Design review of the part built by this model. Coordinates are the model's own, in mm. A direction names the side the tool comes from. Give positions to 0.01 mm unless a question says otherwise; leave off trailing zeros. Write each loop counter-clockwise with the first axis right and the second up, starting at its lowest first coordinate (ties: lowest second). Pieces come first, ordered by that corner, then holes. Notation, with made-up numbers: (85, 67.5) -> (91, 67.5) arc R36 cw to (91, 105.5) -> close; hole circle Ø9 at (37.5, 78). An arc over 180 degrees is marked (long way). Answer as a JSON object with one key per item and string values.
```python
from build123d import *

# Parameters (mm, degrees)
EXTRUDE_1_DEPTH     = 3
SKETCH_2_R          = 1.65
CUT_EXTRUDE_1_DEPTH = 4
SKETCH_3_W          = 40
SKETCH_3_H          = 3
EXTRUDE_2_DEPTH     = 20
EXTRUDE_3_DEPTH     = 1.5


with BuildPart() as part:
    # 草图1 → 凸台-拉伸1 (new body)
    with BuildSketch(Plane(origin=(0, 0, 0), x_dir=(0, 0, -1), z_dir=(1, 0, 0))):
        with BuildLine():
            Line((-20, 0), (20, 0))
            Line((20, 0), (20, 3))
            Line((20, 3), (7.638784068, 24.410254038))
            ThreePointArc((7.638784068, 24.410254038), (0, 28.820508076), (-7.638784068, 24.410254038))
            Line((-7.638784068, 24.410254038), (-20, 3))
            Line((-20, 3), (-20, 0))
        make_face()
    extrude(amount=-EXTRUDE_1_DEPTH)

    # 草图2 → 切除-拉伸1 (cut, through all)
    with BuildSketch(Plane(origin=(0, 0, 0), x_dir=(0, 0, -1), z_dir=(1, 0, 0))):
        with Locations((0, 20)):
            Circle(SKETCH_2_R)
    extrude(amount=-CUT_EXTRUDE_1_DEPTH, mode=Mode.SUBTRACT)

    # 草图3 → 凸台-拉伸2 (add)
    with BuildSketch(Plane(origin=(0, 0, 0), x_dir=(0, 0, -1), z_dir=(1, 0, 0))):
        with Locations((0, 1.5)):
            Rectangle(SKETCH_3_W, SKETCH_3_H)
    extrude(amount=EXTRUDE_2_DEPTH)

    # 草图4 → 凸台-拉伸3 (add, symmetric)
    with BuildSketch(Plane.XY):
        Polygon((0, 3), (0, 15), (12, 3), align=None)
    extrude(amount=EXTRUDE_3_DEPTH, both=True)


solid = part.part
```
(1) We need section A-A, the plane z = 0. State the section outline as (x, y) points, then the cut area to 3 significant figures.
Here are the results:
{"outline": "(-3, 0) -> (20, 0) -> (20, 3) -> (12, 3) -> (0, 15) -> (0, 18.35) -> (-3, 18.35) -> close; (-3, 21.65) -> (0, 21.65) -> (0, 28.82) -> (-3, 28.82) -> close", "area": "209 mm²"}
(2) We need section C-C, the plane y = 20. State the section outline as (x, z) points, then the cut area to 3 significant figures.
Here are the results:
{"outline": "(-3, -10.19) -> (0, -10.19) -> (0, -1.65) -> (-3, -1.65) -> close; (-3, 1.65) -> (0, 1.65) -> (0, 10.19) -> (-3, 10.19) -> close", "area": "51.2 mm²"}
(3) For faces 1 (the flat face through (8, 0, 0)), 2 (the flat face through (20, 2, 0)), 3 (the flat face through (3, 6, -1.5)), 4 (the flat face through (3, 6, 1.5)), 5 (the flat face through (0, 16, 0)), list the 3-axis set-ups (+Z, -Z, +X, -X, +Y, -Y) from which the entire face can be reached by the end or side of a thin tool; tool diameter is ignored.
Here are the results:
{"face 1": "+Z, -Z, +X, -X, -Y", "face 2": "+Z, -Z, +X, +Y, -Y", "face 3": "-Z, +X, +Y", "face 4": "+Z, +X, +Y", "face 5": "+X, +Y"}
(4) Clearance check with flat-ended pins moving along their axes: pin 1 (10 mm diameter, centred on x = 0.5, z = 6, fed in from +Y); pin 2 (2 mm diameter, centred on y = 20, z = 7.5, fed in from +X); pin 3 (6 mm diameter, centred on x = 5.5, y = 9, fed in from -Z); pin 4 (2.5 mm diameter, centred on y = 20, z = 0, fed in from -X) (3 decimals). State where each tip first meets the part, or that it passes through.
Here are the results:
{"pin 1": "stops at y = 28.76", "pin 2": "stops at x = 0", "pin 3": "stops at z = -1.5", "pin 4": "passes through"}
(5) For line 1 along X through (y, z) = (11, 11); line 2 along Z through (x, y) = (5.5, 4.5); line 3 along Y through (x, z) = (7.5, -6.5), list the stretches that pass through material, from the lowest coordinate up.
Here are the results:
{"line 1": "x = -3 to 0", "line 2": "z = -1.5 to 1.5", "line 3": "y = 0 to 3"}
(6) We need section D-D, the plane x = 8.75. State the section outline as (y, z) points, then the cut area to 3 significant figures.
Here are the results:
{"outline": "(0, -20) -> (3, -20) -> (3, -1.5) -> (6.25, -1.5) -> (6.25, 1.5) -> (3, 1.5) -> (3, 20) -> (0, 20) -> close", "area": "130 mm²"}
(7) We need section B-B, the plane x = 4. State the section outline as (y, z) points.
Here are the results:
{"outline": "(0, -20) -> (3, -20) -> (3, -1.5) -> (11, -1.5) -> (11, 1.5) -> (3, 1.5) -> (3, 20) -> (0, 20) -> close"}
